Geometry: final body of the model. Coordinates: model frame, mm. Face numbers are marked on the shaded views. A direction names the side the tool comes from. Give positions to 0.01 mm unless a question says otherwise; leave off trailing zeros. Order: outer loops, then holes, each group sorted by start corner. A loop starts at its lowest first (then second) coordinate and runs counter-clockwise, first axis right, second up. Notation, with made-up numbers: (28.25, 46) -> (49.25, 46) arc R23 ccw to (49.25, 65) -> close; hole circle Ø6 at (70, -33). An arc over 180 degrees is marked (long way). One line per question, with ' | ' between items.
from build123d import *

# Parameters (mm, degrees)
FILLET1_R = 2.5


with BuildPart() as part:
    # Sketch1 → Revolve1 (revolve)
    with BuildSketch(Plane(origin=(0, 0, 0), x_dir=(1, 0, 0), z_dir=(0, 1, 0)), mode=Mode.PRIVATE) as revolve1_sk:
        with BuildLine():
            Line((0, 0), (4.5, 0))
            Line((4.5, 0), (4.5, 17))
            Line((4.5, 17), (3.75, 17))
            add(Edge.make_bspline(
                [(0.75, 17), (2.314018429, 12.999424212), (3.75, 17)],
                knots=[0, 0, 0, 1, 1, 1], degree=2))
            Line((0.75, 17), (0, 17))
            Line((0, 17), (0, 0))
        make_face()
    revolve(revolve1_sk.sketch.rotate(Axis((0, 0, 0), (1, 0, 0)), 180), axis=Axis((0, 0, 0), (1, 0, 0)))

    # Sketch2 → Revolve2 (revolve)
    with BuildSketch(Plane(origin=(0, 0, 0), x_dir=(1, 0, 0), z_dir=(0, 1, 0)), mode=Mode.PRIVATE) as revolve2_sk:
        Polygon((0, 8), (-6.812347486, 8), (-10, 8), (-10, 5.9), (-25, 5.9), (-25, 0), (0, 0), align=None)
    revolve(revolve2_sk.sketch.rotate(Axis((-25, 0, 0), (1, 0, 0)), 180), axis=Axis((-25, 0, 0), (1, 0, 0)))

    # Fillet1
    fillet1_edges = [part.edges().sort_by_distance(p)[0] for p in [
        (-25, 0, -5.9),
    ]]
    fillet(fillet1_edges, radius=FILLET1_R)


solid = part.part
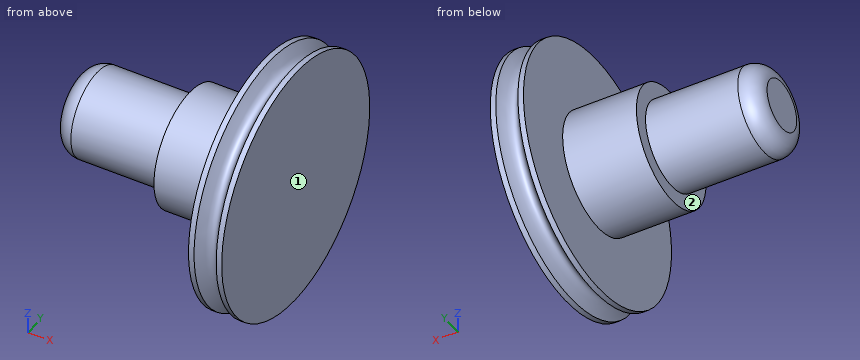
1) Contact query for flat-ended pins moving along their axis: pin 1 Ø5 at (x, y) = (-18.5, 3) entering from +Z; pin 2 Ø8 at (x, y) = (-20, 4) entering from -Z; pin 3 Ø5 at (y, z) = (8.5, 12.5) entering from -X. Output: stop coordinate, or through.
Check result:
pin 1: stops at z = 5.88 | pin 2: stops at z = -5.9 | pin 3: stops at x = 0
2) Section A-A on x = -6.25. Return loops of the section in (y, z), plus the area to 3 significant figures.
Check result:
outline: circle Ø16 at (0, 0) | area: 201 mm^2
3) Material intervals for probe 1 along X at (y, z) = (1, -12.5); probe 2 along Y at (x, z) = (-12, 0); probe 3 along Z at (x, y) = (-15.5, -3.5), sorted ascending. Write a range as from..to.
Check result:
probe 1: x = 0..4.5 | probe 2: y = -5.9..5.9 | probe 3: z = -4.75..4.75
4) Section B-B on x = -10.5. Return loops of the section in (y, z).
Check result:
outline: circle Ø11.8 at (0, 0)
5) Set-up query: the marked faces 1 and 2. Return all of +Z, -Z, +X, -X, +Y, -Y with unobstructed straight access to the full face (end or side cutting, diameter ignored); none if empty.
Check result:
face 1: +Z, -Z, +X, +Y, -Y | face 2: -X
